Model file for the job. Use its own axes, mm. Face numbers are marked on the shaded views. A direction names the side the tool comes from. Coordinates: 2 decimals unless noted, no trailing zeros. Order: outer loops, then holes, each group sorted by start corner. A loop starts at its lowest first (then second) coordinate and runs counter-clockwise, first axis right, second up. Notation, with made-up numbers: (-6, 52.5) -> (21, 52.5) arc R17 ccw to (21, 58.5) -> close; hole circle Ø9 at (52.5, 70.25). An arc over 180 degrees is marked (long way). Return JSON: item names as keys, results as strings. Group by question number.
1) Cut at B-B (y = 32). Write the cut outline in (x, z).
2) Cut at D-D (z = 0). Write the cut outline in (x, y), and give its area (3 significant figures).
3) Probe line 1 (X direction, y = 8.5, z = 33.5); line 2 (Y direction, x = -15, z = 21). List the from-to ranges inside material, lowest first.
4) Cut at A-A (x = -16.5). Write the cut outline in (y, z).
5) Flat gauge pins, fed straight in: pin 1 (5 mm diameter, centred on x = -10, y = 17, fed in from -Z); pin 2 (12 mm diameter, centred on x = -20.5, y = 9, fed in from +Z); pin 3 (4 mm diameter, centred on x = 17.5, y = 39.5, fed in from +Z); pin 4 (3 mm diameter, centred on x = 20.5, z = 2.5, fed in from +Y). Where does each tip first touch, or does it go through?
6) Which spindle directions (+Z, -Z, +X, -X, +Y, -Y) get a long thin tool onto all of the face, cutting with end or side? Do the marked faces 5, 6 and 7. Say none if no direction does.
7) Cut at C-C (z = 21). Write the cut outline in (x, y), and give its area (3 significant figures).
8) Pull direction Y, two halves, no side cores. Call the marked faces 1, 2, 3 and 4: +Y half, -Y half, draft (parallel to the pull), parting line (faces both ways), or undercut.
from build123d import *

# Parameters (mm, degrees)
BOSS_EXTRUDE1_DEPTH = 26
RIB9_REACH          = 65.738
SKETCH6_WALL_W      = 172.022520638
SKETCH6_WALL_H      = 9


with BuildPart() as part:
    # Sketch1 → Boss-Extrude1 (new, symmetric)
    with BuildSketch(Plane(origin=(0, 0, 0), x_dir=(0, 0, -1), z_dir=(1, 0, 0))):
        with BuildLine():
            Line((-23, 44.5), (-15, 44.5))
            ThreePointArc((-15, 44.5), (0, 29.5), (15, 44.5))
            Line((15, 44.5), (23, 44.5))
            ThreePointArc((23, 44.5), (17.783419244, 29.914047854), (4.5, 21.944512863))
            Line((4.5, 21.944512863), (4.5, 4.5))
            Line((4.5, 4.5), (37.5, 4.5))
            Line((37.5, 4.5), (37.5, -4.5))
            Line((37.5, -4.5), (-37.5, -4.5))
            Line((-37.5, -4.5), (-37.5, 4.5))
            Line((-37.5, 4.5), (-4.5, 4.5))
            Line((-4.5, 4.5), (-4.5, 21.944512863))
            ThreePointArc((-4.5, 21.944512863), (-17.783419244, 29.914047854), (-23, 44.5))
        make_face()
    extrude(amount=BOSS_EXTRUDE1_DEPTH, both=True)

    # Sketch6 wall → Rib9 (add, up to next)
    with BuildSketch(Plane(origin=(0, 24.5, -30.25), x_dir=(0, -0.940136065162, -0.340799323621), z_dir=(0, 0.340799323621, -0.940136065162)), mode=Mode.PRIVATE) as rib9_sk1:
        Rectangle(SKETCH6_WALL_W, SKETCH6_WALL_H)
    rib9_tool1 = extrude(rib9_sk1.sketch, amount=-RIB9_REACH, mode=Mode.PRIVATE) - part.part
    rib9 = rib9_tool1.solids().sort_by_distance((0, 24.5, -30.25))[0]
    add(rib9)

    # Mirror1: Rib9 across plane
    add(rib9.mirror(Plane.XY))


solid = part.part
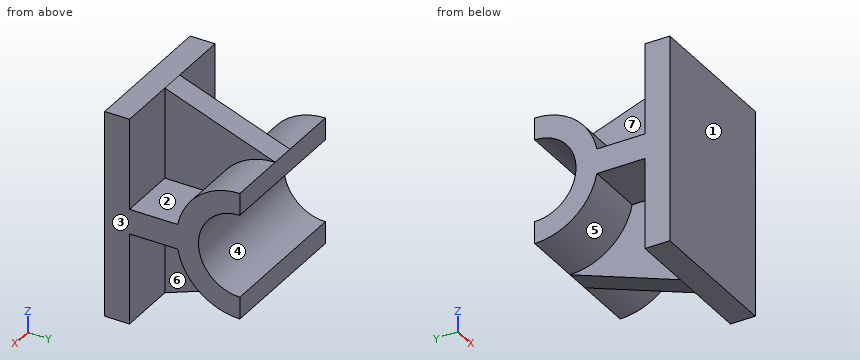
Answers below:
{
 "1": {"outline": "(-26, -19.31) -> (-4.5, -19.31) -> (-4.5, -27.53) -> (4.5, -27.53) -> (4.5, -19.31) -> (26, -19.31) -> (26, -8.29) -> (-26, -8.29) -> close; (-26, 8.29) -> (26, 8.29) -> (26, 19.31) -> (4.5, 19.31) -> (4.5, 27.53) -> (-4.5, 27.53) -> (-4.5, 19.31) -> (-26, 19.31) -> close"},
 "2": {"outline": "(-26, -4.5) -> (26, -4.5) -> (26, 29.5) -> (-26, 29.5) -> close", "area": "1,770 mm^2"},
 "3": {"line 1": "x = -4.5 to 4.5", "line 2": "y = -4.5 to 4.5, 35.12 to 44.5"},
 "4": {"outline": "(-4.5, -37.5) -> (4.5, -37.5) -> (4.5, -4.5) -> (21.94, -4.5) arc R23 ccw to (44.5, -23) -> (44.5, -15) arc R15 cw to (44.5, 15) -> (44.5, 23) arc R23 ccw to (21.94, 4.5) -> (4.5, 4.5) -> (4.5, 37.5) -> (-4.5, 37.5) -> close"},
 "5": {"pin 1": "stops at z = -4.5", "pin 2": "stops at z = 37.5", "pin 3": "stops at z = 22.8", "pin 4": "stops at y = 30.04"},
 "6": {"face 5": "-Z, -X", "face 6": "-Z, +X", "face 7": "+Z, -X"},
 "7": {"outline": "(-26, -4.5) -> (26, -4.5) -> (26, 4.5) -> (4.5, 4.5) -> (4.5, 35.12) -> (26, 35.12) -> (26, 44.5) -> (-26, 44.5) -> (-26, 35.12) -> (-4.5, 35.12) -> (-4.5, 4.5) -> (-26, 4.5) -> close", "area": "1,230 mm^2"},
 "8": {"face 1": "-Y half", "face 2": "undercut", "face 3": "draft", "face 4": "+Y half"}
}
